```python
from build123d import *

# Parameters (mm, degrees)
SKETCH1_W           = 150
SKETCH1_H           = 160
BOSS_EXTRUDE1_DEPTH = 6.35
CUT_EXTRUDE1_REACH  = 111.842


with BuildPart() as part:
    # Sketch1 → Boss-Extrude1 (new body)
    with BuildSketch(Plane.XY):
        Rectangle(SKETCH1_W, SKETCH1_H)
    extrude(amount=BOSS_EXTRUDE1_DEPTH)

    # Sketch2 → Cut-Extrude1 (cut, up to next)
    with BuildSketch(Plane.XY.offset(6.35), mode=Mode.PRIVATE) as cut_extrude1_sk1:
        with BuildLine():
            Line((-24.89, -12), (-24.89, -80))
            Line((-24.89, -80), (24.89, -80))
            Line((24.89, -80), (24.89, -12))
            ThreePointArc((24.89, -12), (0, 12.89), (-24.89, -12))
        make_face()
    cut_extrude1_tool1 = extrude(cut_extrude1_sk1.sketch, amount=-CUT_EXTRUDE1_REACH, mode=Mode.PRIVATE) & part.part
    add(cut_extrude1_tool1.solids().sort_by_distance((0, -36.049464, 6.35))[0], mode=Mode.SUBTRACT)


solid = part.part
```
Work out the finished part from the listing and answer in its coordinate system (mm). A direction names the side the tool comes from. Coordinates: 2 decimals unless noted, no trailing zeros. Write each loop counter-clockwise with the first axis right and the second up, starting at its lowest first coordinate (ties: lowest second). Pieces come first, ordered by that corner, then holes.
Q1. Which of the six approach directions +Z, -Z, +X, -X, +Y, -Y give full straight-line access (tool end or side, diameter ignored) to faces 4 (the face through (-24.89, -46, 3)), 5 (the face through (50, -80, 3))?
Q2. Find the intervals of material crossed by line 1 (X direction, y = -40, z = 5.75); line 2 (X direction, y = -4.5, z = 2.5); line 3 (Y direction, x = 23, z = 5.5), in increasing order.
Q3. Determine the mould class of faces 1 (the face through (-1, 19, 0)), 2 (the face through (-75, -1, 3)), 3 (the face through (0.547, 12.884, 3.219)) for opening direction X: released by +X, released by -X, zero draft, split by the parting line, or undercut.
Q4. A cutting plane is placed at A-A, the plane z = 3.25. Give the vertices of the cut face in (x, y), then the cut area to 3 significant figures.
Q5. A cutting plane is placed at B-B, the plane y = -52.5. Give the vertices of the cut face in (x, z).
Q6. A cutting plane is placed at C-C, the plane x = 0. Give the vertices of the cut face in (y, z), then the cut area to 3 significant figures.
Findings below:
1. face 4: +Z, -Z, -Y
1. face 5: +Z, -Z, +X, -X, -Y
2. line 1: x = -75 to -24.89, 24.89 to 75
2. line 2: x = -75 to -23.73, 23.73 to 75
2. line 3: y = -2.49 to 80
3. face 1: zero draft
3. face 2: released by -X
3. face 3: undercut
4. outline: (-75, -80) - (-24.89, -80) - (-24.89, -12) arc R24.89 cw to (24.89, -12) - (24.89, -80) - (75, -80) - (75, 80) - (-75, 80) - close
4. area: 19,600 mm2
5. outline: (-75, 0) - (-24.89, 0) - (-24.89, 6.35) - (-75, 6.35) - close; (24.89, 0) - (75, 0) - (75, 6.35) - (24.89, 6.35) - close
6. outline: (12.89, 0) - (80, 0) - (80, 6.35) - (12.89, 6.35) - close
6. area: 426 mm2
